from build123d import *

# Parameters (mm, degrees)
F1_DEPTH = 50
F2_W     = 50
F2_H     = 23.9603407681
F3_DEPTH = 60.001
F4_SIZE2 = 10
F4_SIZE  = 20


with BuildPart() as f1:
    # F0 (on Front) → F1 (new body)
    with BuildSketch(Plane.XZ):
        Polygon((-110, 0), (0, 0), (0, 20), (-70, 60), (-110, 60), align=None)
    extrude(amount=-F1_DEPTH)

    # F2 (on face) → F3 (cut, through all)
    with BuildSketch(Plane.XY.offset(60)):
        Polygon((-100, 20), (-100, 0), (-70, 0), (-70, 23.9603407681), (-100, 23.9603407681), align=None)
        with Locations((-45, 11.980170384)):
            Rectangle(F2_W, F2_H)
    extrude(amount=-F3_DEPTH, mode=Mode.SUBTRACT)

    # F4
    f4_edges = [f1.edges().sort_by_distance(p)[0] for p in [
        (-105, 0, 60),
    ]]
    f4_side = f1.faces().sort_by_distance((-92.805245, 32.304762, 60))[0]
    chamfer(f4_edges, length=F4_SIZE, length2=F4_SIZE2, reference=f4_side)


solid = f1.part
Verification items for the finished model (mm, model axes). A direction names the side the tool comes from. Round coordinates to 2 decimals unless told otherwise and drop trailing zeros. Order: outer loops, then holes, each group sorted by start corner. A loop starts at its lowest first (then second) coordinate and runs counter-clockwise, first axis right, second up.
1. Thickness scan on L1, parallel to Y at x = -64.5, z = 34.5; L2, parallel to X at y = 5, z = 14; L3, parallel to X at y = 15, z = 22. Record the ranges inside material, lowest first.
Final values:
L1: y = 23.96 to 50
L2: x = -110 to -100, -20 to 0
L3: x = -110 to -100, -20 to -3.5
2. Section check B-B on z = 26.5. Record the cut outline in (x, y) (3 decimals), then the cut area to 3 significant figures.
Final values:
outline: (-110, 0) - (-100, 0) - (-100, 23.96) - (-20, 23.96) - (-20, 0) - (-11.375, 0) - (-11.375, 50) - (-110, 50) - close
area: 3,010 mm2
3. Release check for a two-part mould opening along X. For faces 1 (the flat face through (-100, 12, 30)), 2 (the flat face through (-56, 30, 0)), 3 (the flat face through (0, 25, 10)) record: +X half, -X half, draft (parallel to the pull), parting line (faces both ways), or undercut.
Final values:
face 1: undercut
face 2: draft
face 3: +X half
4. Section check D-D on x = -87.5. Record the cut outline in (y, z).
Final values:
outline: (23.96, 0) - (50, 0) - (50, 60) - (23.96, 60) - close
5. Go/stop test with flat-tipped pins: P1, Ø10, axis at x = -22.5, y = 28, coming from the +Z side; P2, Ø6, axis at y = 30.5, z = 30.5, coming from the +X side (3 decimals); P3, Ø2, axis at x = -58.5, z = 29.5, coming from the -Y side; P4, Ø12, axis at x = -34.5, y = 24, coming from the -Z side. Record where each tip stops, or that it passes through.
Final values:
P1: stops at z = 35.71
P2: stops at x = -13.125
P3: stops at y = 23.96
P4: stops at z = 0
6. Section check A-A on y = 16. Record the cut outline in (x, z), then the cut area to 3 significant figures.
Final values:
outline: (-110, 0) - (-100, 0) - (-100, 58) - (-110, 58) - close; (-20, 0) - (0, 0) - (0, 20) - (-20, 31.43) - close
area: 1,090 mm2
7. Section check C-C on y = 45. Record the cut outline in (x, z).
Final values:
outline: (-110, 0) - (0, 0) - (0, 20) - (-70, 60) - (-110, 60) - close
8. Access from +Z, -Z, +X, -X, +Y, -Y to the whole of each face (thin tool, end or side, straight path). Record for faces 4 (the flat face through (-20, 12, 16)), 5 (the flat face through (-10, 0, 12)).
Final values:
face 4: +Z, -Z, -Y
face 5: +Z, -Z, +X, -X, -Y
